from build123d import *

# Parameters (mm, degrees)
SKETCH2_R          = 1.397
CUT_EXTRUDE1_DEPTH = 9.4328


with BuildPart() as part:
    # Sketch1 → Revolve1 (revolve)
    with BuildSketch(Plane.XY):
        Polygon((0, 0), (0, 2.159), (1.337955167, 2.159), (1.337955167, 3.302), (0, 3.302), (0, 4.064), (3.7338, 4.064), (3.7338, 3.302), (2.099955167, 3.302), (2.099955167, 2.159), (8.4328, 2.159), (8.4328, 0), align=None)
    revolve(axis=Axis((0, 0, 0), (1, 0, 0)))

    # Sketch2 → Cut-Extrude1 (cut, through all)
    with BuildSketch(Plane.ZY):
        Circle(SKETCH2_R)
    extrude(amount=-CUT_EXTRUDE1_DEPTH, mode=Mode.SUBTRACT)

    # Sketch3 → Revolve2 (revolve)
    with BuildSketch(Plane.XY):
        with BuildLine():
            Line((8.4328, 2.159), (7.1628, 2.159))
            ThreePointArc((7.1628, 2.159), (7.7978, 2.351594416), (8.4328, 2.159))
        make_face()
    revolve(axis=Axis((0, 0, 0), (1, 0, 0)))


solid = part.part
Geometry check sheet. Reference: the model listing, model coordinates, mm. A direction names the side the tool comes from. Give positions to 0.01 mm unless a question says otherwise; leave off trailing zeros. Order: outer loops, then holes, each group sorted by start corner. A loop starts at its lowest first (then second) coordinate and runs counter-clockwise, first axis right, second up.
1) Cross-section at B-B (x = 2.25). Record the boundary of the cut face in (y, z).
Results are:
outline: circle Ø8.13 at (0, 0); circle Ø4.32 at (0, 0); hole circle Ø6.6 at (0, 0); hole circle Ø2.79 at (0, 0)
2) Draft check along Z on faces 1 (the flat face through (0, 2, 3)), 2 (the flat face through (2.1, -0.8, -2.2)), 3 (the cylindrical face through (1.893, -0.881, -3.967)), 4 (the cylindrical face through (0.66, 3.05, -1.26)). Enter one of: released by +Z, released by -Z, zero draft, split by the parting line, or undercut.
Results are:
face 1: zero draft
face 2: undercut
face 3: split by the parting line
face 4: undercut
3) Cross-section at D-D (x = 5.5). Record the boundary of the cut face in (y, z).
Results are:
outline: circle Ø4.32 at (0, 0); hole circle Ø2.79 at (0, 0)
4) Gauge pin test, flat ends, axial feed: pin 1 (3.5 mm diameter, centred on y = 0, z = 0, fed in from -X); pin 2 (4 mm diameter, centred on x = 7.5, z = 0.5, fed in from -Y). Record the tip position at first contact, or that the pin passes through.
Results are:
pin 1: stops at x = 0
pin 2: stops at y = -2.35
5) Tool access check on faces 5 (the cylindrical face through (4.67, -0.28, 2.14)), 6 (the flat face through (1.338, 0.8, -2.2)), 7 (the flat face through (3.734, -2, 3)). Record the directions out of +Z, -Z, +X, -X, +Y, -Y that give a thin tool (end or side, any length) a straight path to the whole face; none if there is none.
Results are:
face 5: none
face 6: -X
face 7: +X
6) Cross-section at A-A (y = 0). Record the boundary of the cut face in (x, z), then the cut area to 3 significant figures.
Results are:
outline: (0, -4.06) - (3.73, -4.06) - (3.73, -3.3) - (2.1, -3.3) - (2.1, -2.16) - (7.16, -2.16) arc R1.14 ccw to (8.43, -2.16) - (8.43, -1.4) - (0, -1.4) - (0, -2.16) - (1.34, -2.16) - (1.34, -3.3) - (0, -3.3) - close; (0, 1.4) - (8.43, 1.4) - (8.43, 2.16) arc R1.14 ccw to (7.16, 2.16) - (2.1, 2.16) - (2.1, 3.3) - (3.73, 3.3) - (3.73, 4.06) - (0, 4.06) - (0, 3.3) - (1.34, 3.3) - (1.34, 2.16) - (0, 2.16) - close
area: 20.6 mm2
7) Material ranges on probe 1 along X at (y, z) = (-1.75, 1.75); probe 2 along X at (y, z) = (-1.75, 3.5); probe 3 along Y at (x, z) = (0.5, -2.25), recorded low to high.
Results are:
probe 1: x = 1.34 to 2.1
probe 2: x = 0 to 3.73
probe 3: y = -3.38 to -2.42, 2.42 to 3.38
